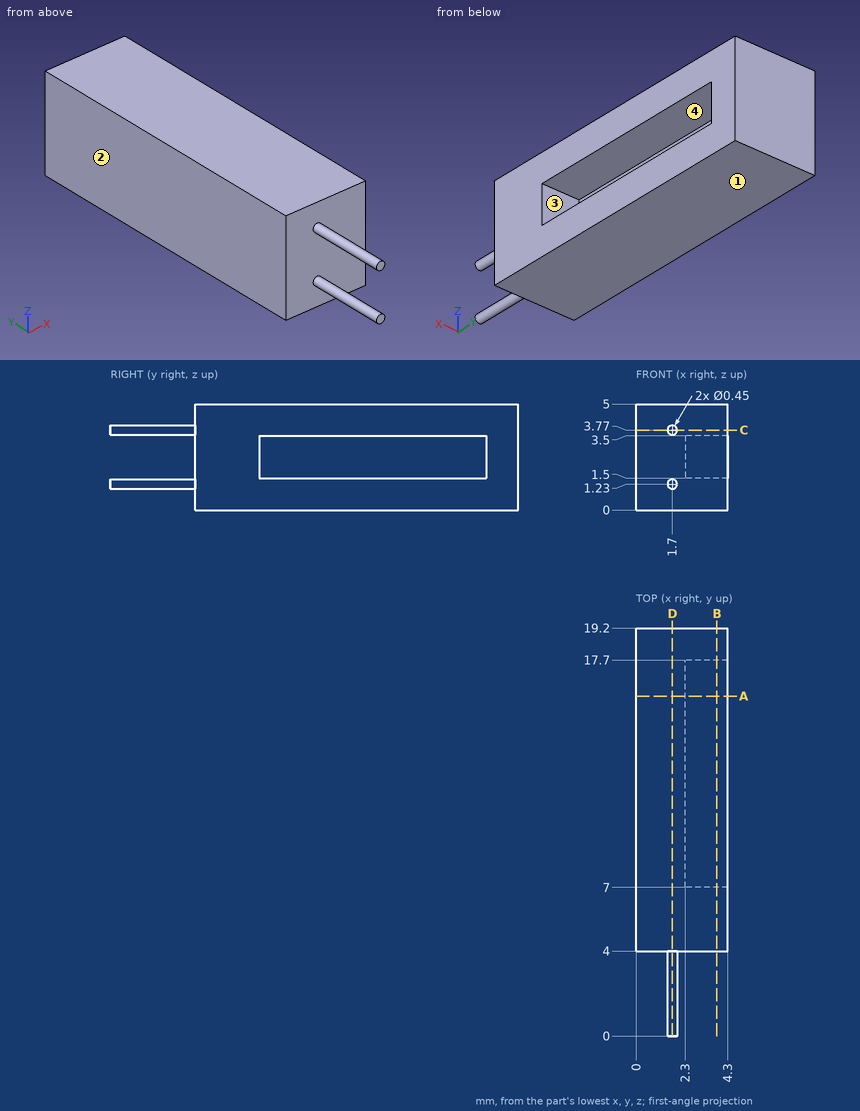
For this review, use the dimensioned drawing (mm, ordinates from the lowest corner) and the shaded views. Coordinates: 2 decimals unless noted, no trailing zeros. Loops run counter-clockwise (first coordinate to the right, second up) from the corner with the lowest first, then second, coordinate; pieces in that order, holes last. Notation, with made-up numbers: (37, -37.5) - (53, -37.5) arc R30 ccw to (53, -2.5) - close; hole circle Ø6 at (66.25, 16.5). An arc over 180 degrees is marked (long way). Use CSV: the item, a comma, the result in double quotes. Start each with the question number.
1) For pin 1 Ø1.6 at (x, z) = (3, 2) entering from -Y, flat-tipped, find the tip position at first contact; note if it passes through.
2) The part is to be moulded in two halves that separate along Z. For the marked faces 1, 2, 3 and 4, say which applies: +Z half, -Z half, draft (parallel to the pull), parting line (faces both ways), or undercut.
3) Consider section A-A on y = 16. Write out the cut boundary in (x, z), then the cut area to 3 significant figures.
4) Wall thickness on L1, parallel to Y at x = 2.55, z = 1.85; L2, parallel to Z at x = 3.1, y = 10.75; L3, parallel to X at y = 12.25, z = 3.25: over which ranges is each line inside the solid? List them lowest first. Write a range as from..to.
5) Consider section C-C on z = 3.77. Write out the cut boundary in (x, y) (3 decimals).
6) Consider section B-B on x = 3.8. Write out the cut boundary in (y, z), then the cut area to 3 significant figures.
7) Consider section D-D on x = 1.7. Write out the cut boundary in (y, z) (3 decimals), then the cut area to 3 significant figures.
Geometry says:
1,pin 1,"y = 4"
2,face 1,"-Z half"
2,face 2,"draft"
2,face 3,"undercut"
2,face 4,"undercut"
3,outline,"(0, 0) - (4.3, 0) - (4.3, 1.5) - (2.3, 1.5) - (2.3, 3.5) - (4.3, 3.5) - (4.3, 5) - (0, 5) - close"
3,area,"17.5 mm^2"
4,L1,"4..7, 17.7..19.2"
4,L2,"0..1.5, 3.5..5"
4,L3,"0..2.3"
5,outline,"(0, 4) - (1.475, 4) - (1.475, 0) - (1.925, 0) - (1.925, 4) - (4.3, 4) - (4.3, 19.2) - (0, 19.2) - close"
6,outline,"(4, 0) - (19.2, 0) - (19.2, 5) - (4, 5) - close; hole (7, 1.5) - (17.7, 1.5) - (17.7, 3.5) - (7, 3.5) - close"
6,area,"54.6 mm^2"
7,outline,"(0, 1.005) - (4, 1.005) - (4, 0) - (19.2, 0) - (19.2, 5) - (4, 5) - (4, 3.995) - (0, 3.995) - (0, 3.545) - (4, 3.545) - (4, 1.455) - (0, 1.455) - close"
7,area,"79.6 mm^2"
